Geometry check sheet. Reference: the model listing, model coordinates, mm. Face numbers are marked on the shaded views. A direction names the side the tool comes from. Give positions to 0.01 mm unless a question says otherwise; leave off trailing zeros. Loops run counter-clockwise (first coordinate to the right, second up) from the corner with the lowest first, then second, coordinate; pieces in that order, holes last. Notation, with made-up numbers: (25.25, -24.75) -> (35.25, -24.75) arc R31 cw to (35.25, 9.25) -> close; hole circle Ø10 at (50.5, 61). An arc over 180 degrees is marked (long way). Answer as a JSON object with one key per item and string values.
from build123d import *

# Parameters (mm, degrees)
SALIENTE_EXTRUIR1_DEPTH = 14
CROQUIS2_W              = 40
CROQUIS2_H              = 3
SALIENTE_EXTRUIR2_DEPTH = 25
CROQUIS3_W              = 11
CROQUIS3_H              = 11
CORTAR_EXTRUIR1_DEPTH   = 12
REDONDEO1_R             = 2.5


with BuildPart() as part:
    # Croquis1 → Saliente-Extruir1 (new body)
    with BuildSketch(Plane(origin=(0, 0, 0), x_dir=(1, 0, 0), z_dir=(0, 1, 0))):
        Polygon((-40, 0), (-40, 25), (0, 25), (0, 0), (3, 0), (3, 28), (-43, 28), (-43, 0), align=None)
    extrude(amount=SALIENTE_EXTRUIR1_DEPTH)

    # Croquis2 → Saliente-Extruir2 (add)
    with BuildSketch(Plane.XY.offset(-25)):
        with Locations((-20, 12.5)):
            Rectangle(CROQUIS2_W, CROQUIS2_H)
    extrude(amount=SALIENTE_EXTRUIR2_DEPTH)

    # Croquis3 → Cortar-Extruir1 (cut)
    with BuildSketch(Plane(origin=(3, 0, 0), x_dir=(0, 0, -1), z_dir=(1, 0, 0))):
        with Locations((19.5, 5.5)):
            Rectangle(CROQUIS3_W, CROQUIS3_H)
    extrude(amount=-CORTAR_EXTRUIR1_DEPTH, mode=Mode.SUBTRACT)

    # Redondeo1
    redondeo1_edges = [part.edges().sort_by_distance(p)[0] for p in [
        (-18.5, 11, -25),
        (3, 14, -14),
        (-20, 14, -28),
        (1.5, 11, -14),
        (-43, 14, -14),
    ]]
    fillet(redondeo1_edges, radius=REDONDEO1_R)


solid = part.part
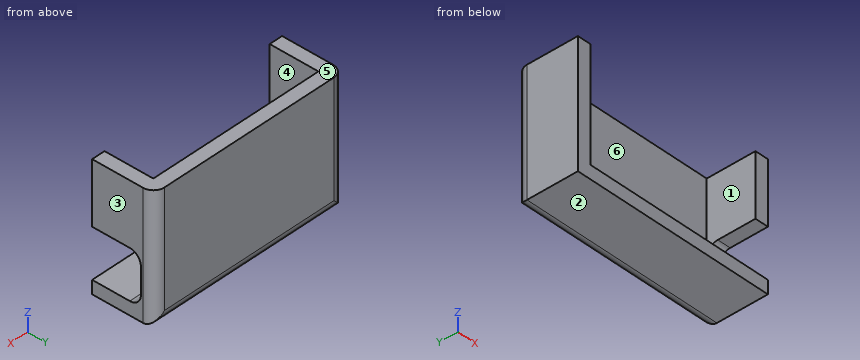
1) Section check B-B on x = -27. Record the cut outline in (y, z).
Geometry check:
{"outline": "(0, -28) -> (11.5, -28) arc R2.5 ccw to (14, -25.5) -> (14, 0) -> (11, 0) -> (11, -22.5) arc R2.5 cw to (8.5, -25) -> (0, -25) -> close"}
2) Tool access check on the marked faces 1 and 2. Record the directions out of +Z, -Z, +X, -X, +Y, -Y that give a thin tool (end or side, any length) a straight path to the whole face; none if there is none.
Geometry check:
{"face 1": "+Z, -Y", "face 2": "-Z, +X, -X, +Y, -Y"}
3) Depth check by flat-ended pin: P1, Ø6, axis at x = -36, z = -12.5, coming from the -Y side. Enter the tip coordinate at first touch or a pass-through.
Geometry check:
{"P1": "stops at y = 11"}
4) Section check D-D on y = 10.5. Record the cut outline in (x, z), plus the area to 3 significant figures.
Geometry check:
{"outline": "(-43, -28) -> (3, -28) -> (3, -24) -> (-40, -24) -> (-40, 0) -> (-43, 0) -> close; (0, -15) -> (3, -15) -> (3, 0) -> (0, 0) -> close", "area": "301 mm2"}
5) Section check C-C on z = -21. Record the cut outline in (x, y), plus the area to 3 significant figures.
Geometry check:
{"outline": "(-43, 0) -> (-40, 0) -> (-40, 11) -> (3, 11) -> (3, 11.5) arc R2.5 ccw to (0.5, 14) -> (-40.5, 14) arc R2.5 ccw to (-43, 11.5) -> close", "area": "168 mm2"}
6) Section check A-A on y = 6.75. Record the cut outline in (x, z).
Geometry check:
{"outline": "(-43, -28) -> (3, -28) -> (3, -25) -> (-40, -25) -> (-40, 0) -> (-43, 0) -> close; (0, -14) -> (3, -14) -> (3, 0) -> (0, 0) -> close"}
7) Draft check along X on the marked faces 3, 4, 5 and 6. Enter one of: pulls with the +X half, pulls with the -X half, needs draft (parallel to the pull), parting line crosses it, or undercut.
Geometry check:
{"face 3": "pulls with the +X half", "face 4": "undercut", "face 5": "needs draft", "face 6": "undercut"}
8) Material ranges on line 1 along X through (y, z) = (2.5, -9.5); line 2 along Y through (x, z) = (-15.5, -15); line 3 along X through (y, z) = (5.5, -16.75), recorded low to high. Write a range as from..to.
Geometry check:
{"line 1": "x = -43..-40, 0..3", "line 2": "y = 11..14", "line 3": "x = -43..-40"}
